Can you work these out from the model? Positions are in its coordinate system, mm. A direction names the side the tool comes from. Give positions to 0.01 mm unless a question says otherwise; leave off trailing zeros. Write each loop counter-clockwise with the first axis right and the second up, starting at its lowest first coordinate (ties: lowest second). Pieces come first, ordered by that corner, then holes. Notation, with made-up numbers: M 78.5,89 L 128.5,89 A5 ccw 128.5,95 Z; hole C 59,-6 d7. An arc over 180 degrees is marked long. Write each question's results on one line, items separated by ' | '.
from build123d import *

# Parameters (mm, degrees)
SZKIC1_W                    = 100
SZKIC1_H                    = 80
SZKIC1_R                    = 3.55
SZKIC1_R_2                  = 2.05
SZKIC1_R_3                  = 2.55
SZKIC1_R_4                  = 12.5
SZKIC1_W_2                  = 20.5
SZKIC1_H_2                  = 40.5
DODANIE_WYCI_GNI_CIE1_DEPTH = 3


with BuildPart() as part:
    # Szkic1 → Dodanie-wyciągnięcie1 (new body)
    with BuildSketch(Plane(origin=(0, 0, 0), x_dir=(1, 0, 0), z_dir=(0, 1, 0))):
        with Locations((11.336719097, -8.838965942)):
            Rectangle(SZKIC1_W, SZKIC1_H)
        with Locations(Location((44.775116298, -18.788965942, 0), (0, 0, 270))):
            Circle(SZKIC1_R, mode=Mode.SUBTRACT)
        with Locations(Location((28.775116298, -32.588965942, 0), (0, 0, 270))):
            Circle(SZKIC1_R_2, mode=Mode.SUBTRACT)
        with Locations(Location((18.775116298, -32.588965942, 0), (0, 0, 270))):
            Circle(SZKIC1_R_2, mode=Mode.SUBTRACT)
        with Locations(Location((28.775116298, 14.911034058, 0), (0, 0, 270))):
            Circle(SZKIC1_R_2, mode=Mode.SUBTRACT)
        with Locations(Location((18.775116298, 14.911034058, 0), (0, 0, 270))):
            Circle(SZKIC1_R_2, mode=Mode.SUBTRACT)
        with Locations(Location((-20.268770099, -13.743104788, 0), (0, 0, 270))):
            Circle(SZKIC1_R_3, mode=Mode.SUBTRACT)
        with Locations(Location((5.231229901, -13.743104788, 0), (0, 0, 270))):
            Circle(SZKIC1_R_3, mode=Mode.SUBTRACT)
        with Locations(Location((5.231229901, 11.756895212, 0), (0, 0, 270))):
            Circle(SZKIC1_R_3, mode=Mode.SUBTRACT)
        with Locations(Location((-20.268770099, 11.756895212, 0), (0, 0, 270))):
            Circle(SZKIC1_R_3, mode=Mode.SUBTRACT)
        with Locations(Location((-7.518770099, -0.993104788, 0), (0, 0, 270))):
            Circle(SZKIC1_R_4, mode=Mode.SUBTRACT)
        with Locations((23.775116298, -8.838965942)):
            Rectangle(SZKIC1_W_2, SZKIC1_H_2, mode=Mode.SUBTRACT)
    extrude(amount=DODANIE_WYCI_GNI_CIE1_DEPTH)


solid = part.part
Item 1: I want a section at D-D, the plane x = 1. Please give me the cut outline in (y, z), and give its area (3 significant figures).
Geometry says:
outline: M 0,-31.16 L 3,-31.16 L 3,-8.15 L 0,-8.15 Z; M 0,10.14 L 3,10.14 L 3,48.84 L 0,48.84 Z | area: 185 mm2
Item 2: Thinking about a two-plate mould opening in Z: for faces 3 (the face through (18.87, 1.48, -16.96)), 4 (the face through (-38.663, 1, 9)), 5 (the face through (11, 1, 48.839)), which applies, +Z half, -Z half, draft (parallel to the pull), parting line (faces both ways), or undercut?
Geometry says:
face 3: undercut | face 4: draft | face 5: +Z half
Item 3: If I drill on line 1 (X direction, y = 2.15, z = 25); line 2 (X direction, y = 1.55, z = 5.5); line 3 (X direction, y = 1.55, z = -8), over which ranges is the centre line in solid material (lowest first)? Write a range as from..to.
Geometry says:
line 1: x = -38.66..13.53, 34.03..61.34 | line 2: x = -38.66..-19.18, 4.14..13.53, 34.03..61.34 | line 3: x = -38.66..-16.2, 1.16..13.53, 34.03..61.34
Item 4: I want a section at A-A, the plane x = 15. Please give me the cut outline in (y, z).
Geometry says:
outline: M 0,-31.16 L 3,-31.16 L 3,-11.41 L 0,-11.41 Z; M 0,29.09 L 3,29.09 L 3,48.84 L 0,48.84 Z
Item 5: I want a section at B-B, the plane y = 1.3. Give the number of separate pieces and of enclosed holes in the cut face, and give its area (3 significant figures).
Geometry says:
separate pieces: 1 | enclosed holes: 11 | area: 6,500 mm2
Item 6: I'm going to push a flat-ended pin straight in: pin 1 (3.5 mm diameter, centred on x = 28.78, z = -14.91, fed in from +Y). Where does the tip first touch, or does it pass through?
Geometry says:
pin 1: passes through
Item 7: For faces 1 (the face through (11, 3, 8)), 2 (the face through (24, 1, 29.089)), which set-ups out of +Z, -Z, +X, -X, +Y, -Y let a thin tool reach every point of the face, with its end or its side?
Geometry says:
face 1: +Z, -Z, +X, -X, +Y | face 2: +Y, -Y
Item 8: I want a section at C-C, the plane z = -4. Please give me the cut outline in (x, y), and give its area (3 significant figures).
Geometry says:
outline: M -38.66,0 L -18.98,0 L -18.98,3 L -38.66,3 Z; M 3.94,0 L 13.53,0 L 13.53,3 L 3.94,3 Z; M 34.03,0 L 61.34,0 L 61.34,3 L 34.03,3 Z | area: 170 mm2
